from build123d import *

# Parameters (mm, degrees)
BOSS_EXTRUDE1_DEPTH                                 = 5
SKETCH2_R                                           = 2.75
CUT_EXTRUDE1_DEPTH                                  = 3
CBORE_FOR_M3_HEX_SOCKET_HEAD_CAP_SCREW1_D           = 3.4
CBORE_FOR_M3_HEX_SOCKET_HEAD_CAP_SCREW1_CBORE_D     = 6.5
CBORE_FOR_M3_HEX_SOCKET_HEAD_CAP_SCREW1_CBORE_DEPTH = 3.5
CHAMFER1_SIZE                                       = 0.5


with BuildPart() as part:
    # Sketch1 → Boss-Extrude1 (new body)
    with BuildSketch(Plane(origin=(0, 0, 0), x_dir=(1, 0, 0), z_dir=(0, 1, 0))):
        with BuildLine():
            Line((-7.5, 4.25), (7.5, 4.25))
            ThreePointArc((7.5, 4.25), (11.75, 0), (7.5, -4.25))
            Line((7.5, -4.25), (-7.5, -4.25))
            ThreePointArc((-7.5, -4.25), (-11.75, 0), (-7.5, 4.25))
        make_face()
    extrude(amount=BOSS_EXTRUDE1_DEPTH)

    # Sketch2 → Cut-Extrude1 (cut)
    with BuildSketch(Plane(origin=(0, 5, 0), x_dir=(1, 0, 0), z_dir=(0, 1, 0))):
        with Locations(Location((0, 0, 0), (0, 0, 270))):
            Circle(SKETCH2_R)
    extrude(amount=-CUT_EXTRUDE1_DEPTH, mode=Mode.SUBTRACT)

    # CBORE for M3 Hex Socket Head Cap Screw1 (through all)
    with Locations(Plane(origin=(0, 5, 0), x_dir=(1, 0, 0), z_dir=(0, 1, 0))):
        with Locations((-7.5, 0), (7.5, 0)):
            CounterBoreHole(CBORE_FOR_M3_HEX_SOCKET_HEAD_CAP_SCREW1_D / 2, CBORE_FOR_M3_HEX_SOCKET_HEAD_CAP_SCREW1_CBORE_D / 2, CBORE_FOR_M3_HEX_SOCKET_HEAD_CAP_SCREW1_CBORE_DEPTH)

    # Chamfer1
    chamfer1_edges = [part.edges().sort_by_distance(p)[0] for p in [
        (0, 5, -2.75),
    ]]
    chamfer(chamfer1_edges, length=CHAMFER1_SIZE)


solid = part.part
Source: CAD feature listing. Evaluate the final solid. Frame: model axes, mm. A direction names the side the tool comes from. Give positions to 0.01 mm unless a question says otherwise; leave off trailing zeros. Order: outer loops, then holes, each group sorted by start corner. A loop starts at its lowest first (then second) coordinate and runs counter-clockwise, first axis right, second up. Notation, with made-up numbers: (-12.5, -16) -> (41.5, -16) arc R18 cw to (41.5, 18) -> close; hole circle Ø11 at (37.5, -14.75). An arc over 180 degrees is marked (long way). Write item = value, one per line.
Item 1: Section query A-A (z = 0). Output: boundary loops of the cut face in (x, y), then the cut area to 4 significant figures.
Check result:
outline = (-11.75, 0) -> (-9.2, 0) -> (-9.2, 1.5) -> (-10.75, 1.5) -> (-10.75, 5) -> (-11.75, 5) -> close; (-5.8, 0) -> (5.8, 0) -> (5.8, 1.5) -> (4.25, 1.5) -> (4.25, 5) -> (3.25, 5) -> (2.75, 4.5) -> (2.75, 2) -> (-2.75, 2) -> (-2.75, 4.5) -> (-3.25, 5) -> (-4.25, 5) -> (-4.25, 1.5) -> (-5.8, 1.5) -> close; (9.2, 0) -> (11.75, 0) -> (11.75, 5) -> (10.75, 5) -> (10.75, 1.5) -> (9.2, 1.5) -> close
area = 45.05 mm²
Item 2: Section query B-B (x = 0). Output: boundary loops of the cut face in (y, z).
Check result:
outline = (0, -4.25) -> (5, -4.25) -> (5, -3.25) -> (4.5, -2.75) -> (2, -2.75) -> (2, 2.75) -> (4.5, 2.75) -> (5, 3.25) -> (5, 4.25) -> (0, 4.25) -> close
Item 3: Section query D-D (x = -8.25). Output: boundary loops of the cut face in (y, z), then the cut area to 3 significant figures.
Check result:
outline = (0, -4.18) -> (5, -4.18) -> (5, -3.16) -> (1.5, -3.16) -> (1.5, -1.53) -> (0, -1.53) -> close; (0, 1.53) -> (1.5, 1.53) -> (1.5, 3.16) -> (5, 3.16) -> (5, 4.18) -> (0, 4.18) -> close
area = 15.1 mm²
Item 4: Ray query, probe 1 along X at (y, z) = (3, 1.25); probe 2 along X at (y, z) = (3, -2.5); probe 3 along X at (y, z) = (3.9, 3). Return the intervals inside material, ascending.
Check result:
probe_1 = -11.56 to -10.5, -4.5 to -2.45, 2.45 to 4.5, 10.5 to 11.56
probe_2 = -10.94 to -9.58, -5.42 to -1.15, 1.15 to 5.42, 9.58 to 10.94
probe_3 = -10.51 to -8.75, -6.25 to 6.25, 8.75 to 10.51
Item 5: Set-up query: faces 4 (the face through (4.253, 3.274, -0.143)), 5 (the face through (-6.15, 0.74, 1.03)). Return all of +Z, -Z, +X, -X, +Y, -Y with unobstructed straight access to the full face (end or side cutting, diameter ignored); none if empty.
Check result:
face_4 = +Y
face_5 = +Y, -Y
Item 6: Section query C-C (y = 3.65). Output: boundary loops of the cut face in (x, z).
Check result:
outline = (-7.5, -4.25) -> (7.5, -4.25) arc R4.25 ccw to (7.5, 4.25) -> (-7.5, 4.25) arc R4.25 ccw to start; hole circle Ø6.5 at (-7.5, 0); hole circle Ø5.5 at (0, 0); hole circle Ø6.5 at (7.5, 0)
Item 7: Mould query, pull axis Z, two halves, no side actions, for faces 1 (the face through (0, 2, 0)), 2 (the face through (0, 0, 0)), 3 (the face through (0, 2, -4.25)). Classes: +Z half, -Z half, draft (parallel to the pull), parting line (faces both ways), or undercut.
Check result:
face_1 = undercut
face_2 = draft
face_3 = -Z half
Item 8: Contact query for flat-ended pins moving along their axis: pin 1 (3 mm diameter, centred on x = 9, z = -0.5, fed in from +Y); pin 2 (2 mm diameter, centred on y = 4, z = 1, fed in from -X); pin 3 (3 mm diameter, centred on x = -7.5, z = 0, fed in from +Y). Output: stop coordinate, or through.
Check result:
pin_1 = 1.5
pin_2 = -11.75
pin_3 = through
